Could you check a few things on this drawing? It's one solid part, dimensions in mm from its lowest x, y, z. A direction names the side the tool comes from. Give positions to 0.01 mm unless a question says otherwise; leave off trailing zeros. Loops run counter-clockwise (first coordinate to the right, second up) from the corner with the lowest first, then second, coordinate; pieces in that order, holes last. Notation, with made-up numbers: (58, -7) - (97, -7) arc R19 cw to (97, 28) - close; hole circle Ø3 at (18.5, 40). An arc over 180 degrees is marked (long way). Use a Markdown table: item, result.
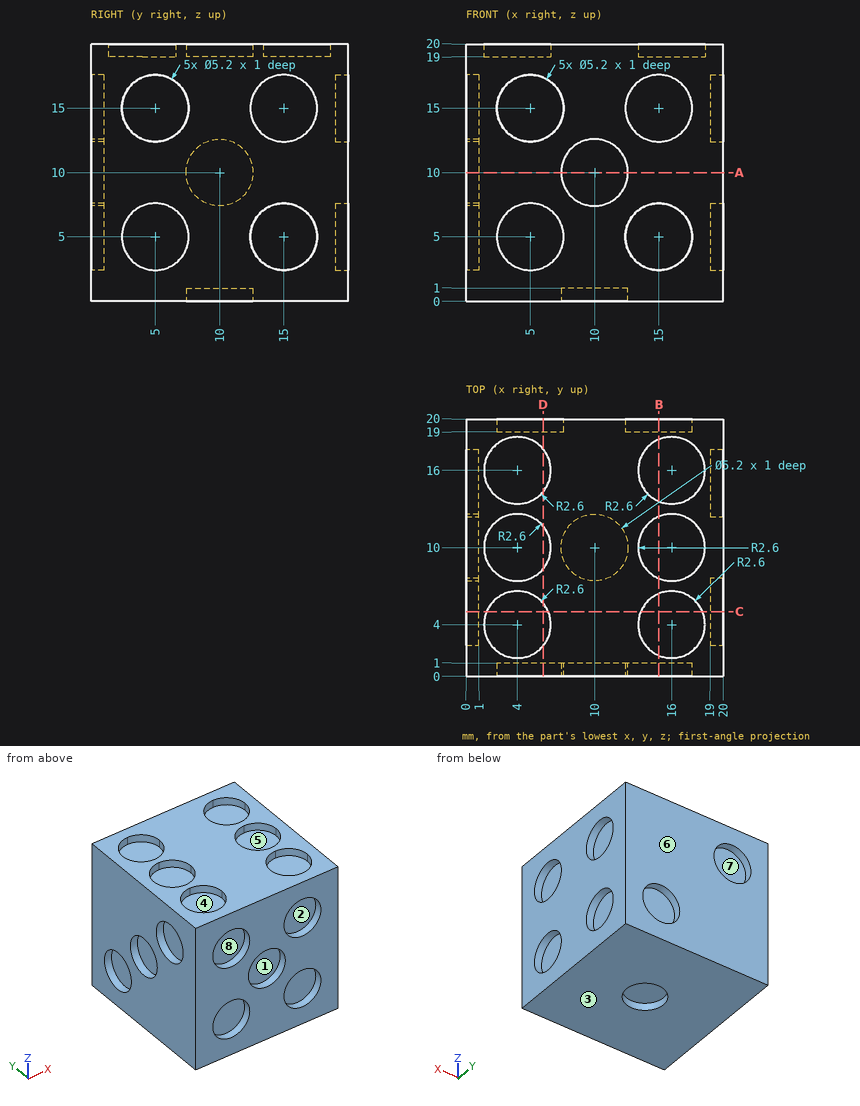
(1) Suppose I cut it at C-C on y = 5. Write out the boundary of the cut face in (x, z).
A:
| item | result |
|---|---|
| outline | (0, 0) - (20, 0) - (20, 2.4) - (19, 2.4) - (19, 7.6) - (20, 7.6) - (20, 12.4) - (19, 12.4) - (19, 17.6) - (20, 17.6) - (20, 20) - (18.4, 20) - (18.4, 19) - (13.6, 19) - (13.6, 20) - (6.4, 20) - (6.4, 19) - (1.6, 19) - (1.6, 20) - (0, 20) - (0, 17.6) - (1, 17.6) - (1, 12.4) - (0, 12.4) - close |
(2) Will these pins go through, and if not, where does the flat tip stop? pin 1 (3 mm diameter, centred on y = 5, z = 15, fed in from +X); pin 2 (1.6 mm diameter, centred on x = 5.5, z = 14.5, fed in from +Y); pin 3 (3 mm diameter, centred on x = 15, z = 5, fed in from -Y); pin 4 (10 mm diameter, centred on x = 13, z = 15.5, fed in from -Y).
A:
| item | result |
|---|---|
| pin 1 | x = 19 |
| pin 2 | y = 19 |
| pin 3 | y = 1 |
| pin 4 | y = 0 |
(3) If I drill on line 1 (Z direction, x = 15, y = 0.6); line 2 (Z direction, x = 0.3, y = 10); line 3 (Z direction, x = 2.25, y = 4.5), over which ranges is the centre line in solid material (lowest first)?
A:
| item | result |
|---|---|
| line 1 | 0 to 2.4, 7.6 to 12.4, 17.6 to 20 |
| line 2 | 0 to 7.4, 12.6 to 20 |
| line 3 | 0 to 19 |
(4) On a 3-axis mill with a long thin cutter (end or side, diameter ignored), from which of +Z, -Z, +X, -X, +Y, -Y can I reach the whole of each face in a straight line? I mean the marked faces 5, 6, 7 and 8. Say none if no direction works.
A:
| item | result |
|---|---|
| face 5 | +Z |
| face 6 | +Z, -Z, +X, -X, +Y |
| face 7 | +Y |
| face 8 | -Y |
(5) Suppose I cut it at A-A on z = 10. Write out the boundary of the cut face in (x, y), plus the area to 3 significant figures.
A:
| item | result |
|---|---|
| outline | (0, 0) - (7.4, 0) - (7.4, 1) - (12.6, 1) - (12.6, 0) - (20, 0) - (20, 20) - (0, 20) - (0, 12.6) - (1, 12.6) - (1, 7.4) - (0, 7.4) - close |
| area | 390 mm2 |
(6) We'd pull the mould along Z, two halves only. Please class the marked faces 1, 2, 3 and 4: pulls with the +Z half, pulls with the -Z half, needs draft (parallel to the pull), parting line crosses it, or undercut.
A:
| item | result |
|---|---|
| face 1 | undercut |
| face 2 | undercut |
| face 3 | pulls with the -Z half |
| face 4 | pulls with the +Z half |
(7) Suppose I cut it at D-D on x = 6. Write out the boundary of the cut face in (y, z).
A:
| item | result |
|---|---|
| outline | (0, 0) - (20, 0) - (20, 12.6) - (19, 12.6) - (19, 17.4) - (20, 17.4) - (20, 20) - (17.66, 20) - (17.66, 19) - (14.34, 19) - (14.34, 20) - (11.66, 20) - (11.66, 19) - (8.34, 19) - (8.34, 20) - (5.66, 20) - (5.66, 19) - (2.34, 19) - (2.34, 20) - (0, 20) - (0, 17.4) - (1, 17.4) - (1, 12.6) - (0, 12.6) - (0, 7.4) - (1, 7.4) - (1, 2.6) - (0, 2.6) - close |
(8) Suppose I cut it at B-B on x = 15. Write out the boundary of the cut face in (y, z).
A:
| item | result |
|---|---|
| outline | (0, 0) - (20, 0) - (20, 2.4) - (19, 2.4) - (19, 7.6) - (20, 7.6) - (20, 20) - (18.4, 20) - (18.4, 19) - (13.6, 19) - (13.6, 20) - (12.4, 20) - (12.4, 19) - (7.6, 19) - (7.6, 20) - (6.4, 20) - (6.4, 19) - (1.6, 19) - (1.6, 20) - (0, 20) - (0, 17.6) - (1, 17.6) - (1, 12.4) - (0, 12.4) - (0, 7.6) - (1, 7.6) - (1, 2.4) - (0, 2.4) - close |
